For this review, take the finished solid that the model builds, in its own axes (mm). A direction names the side the tool comes from. Give positions to 0.01 mm unless a question says otherwise; leave off trailing zeros. Loops run counter-clockwise (first coordinate to the right, second up) from the corner with the lowest first, then second, coordinate; pieces in that order, holes last.
Autodesk Inventor part; units mm, degrees
ref_plane "YZ Plane" through (0, 0, 0) normal (1, 0, 0) x (0, 1, 0)
ref_plane "XZ Plane" through (0, 0, 0) normal (0, 1, 0) x (-1, 0, 0)
ref_plane "XY Plane" through (0, 0, 0) normal (0, 0, 1) x (1, 0, 0)
sketch "Sketch1" plane through (0, 0, 0) normal (0, 0, 1) x (1, 0, 0)
  line L0 (1.5, 0) -> (25.67, 0)
  line L1 (27.17, 1.5) -> (27.17, 38.5)
  line L2 (25.67, 40) -> (1.5, 40)
  line L3 (0, 38.5) -> (0, 1.5)
  arc A0 (1.5, 40) -> (0, 38.5) centre (1.5, 38.5) ccw
  arc A1 (27.17, 38.5) -> (25.67, 40) centre (25.67, 38.5) ccw
  arc A2 (25.67, 0) -> (27.17, 1.5) centre (25.67, 1.5) ccw
  arc A3 (0, 1.5) -> (1.5, 0) centre (1.5, 1.5) ccw
  point P0 (0, 0)
  point P1 (27.17, 40)
  point P2 (0, 40)
  dimension "d0" = 40
  dimension "d1" = 27.17
  dimension "d2" = 1.5
extrude "Extrusion1" add sketch "Sketch1" along normal blind 1.6
sketch "Sketch2" plane through (0, 0, 1.6) normal (0, 0, 1) x (1, 0, 0)
  line L0 (25.67, 40) -> (1.5, 40)
  line L1 (6, 40) -> (21, 40)
  line L2 (21, 40) -> (21, 25)
  line L3 (21, 25) -> (6, 25)
  line L4 (6, 25) -> (6, 40)
  line L5 (0, 38.5) -> (0, 1.5)
  line L6 (5.5, 17.5) -> (21.8, 17.5)
  line L7 (21.8, 17.5) -> (21.8, 11.8)
  line L8 (21.8, 11.8) -> (5.5, 11.8)
  line L9 (5.5, 11.8) -> (5.5, 17.5)
  line L10 (1.5, 0) -> (25.67, 0)
  line L11 (27.17, 1.5) -> (27.17, 38.5)
  line L12 (27.17, 12.8) -> (23.17, 12.8)
  line L13 (23.17, 12.8) -> (23.17, 8.8)
  line L14 (23.17, 8.8) -> (27.17, 8.8)
  line L15 (27.17, 8.8) -> (27.17, 12.8)
  point P0 (0, 0)
  dimension "d5" = 15
  dimension "d6" = 15
  dimension "d7" = 6
  dimension "d8" = 5.7
  dimension "d9" = 16.3
  dimension "d10" = 5.5
  dimension "d11" = 11.8
  dimension "d12" = 4
  dimension "d13" = 4
  dimension "d14" = 8.8
extrude "Extrusion2" add sketch "Sketch2" along normal blind 2 contours L2 L3 L4 L0
extrude "Extrusion3" add sketch "Sketch2" along normal blind 2 contours L6 L7 L8 L9
extrude "Extrusion4" add sketch "Sketch2" along normal blind 1 contours L14 L13 L12 L11
sketch "Sketch3" plane through (0, 0, 3.6) normal (0, 0, 1) x (1, 0, 0)
  line L0 (10.37, 36.1) -> (18.47, 36.1)
  line L1 (18.47, 36.1) -> (18.47, 28)
  line L2 (18.47, 28) -> (10.37, 28)
  line L3 (10.37, 28) -> (10.37, 36.1)
  line L4 (25.67, 40) -> (21, 40)
  line L5 (27.17, 12.8) -> (27.17, 38.5)
  point P0 (0, 0)
  dimension "d21" = 8.1
  dimension "d22" = 8.1
  dimension "d23" = 3.9
  dimension "d24" = 8.7
extrude "Extrusion5" add sketch "Sketch3" along normal blind 2.2
sketch "Sketch4" plane through (0, 0, 5.8) normal (0, 0, 1) x (1, 0, 0)
  circle A0 centre (14.42, 32.05) radius 3.9
  circle A1 centre (14.42, 32.05) radius 4.05
  line L0 (18.47, 36.1) -> (10.37, 36.1)
  line L1 (18.47, 28) -> (18.47, 36.1)
  point P0 (0, 0)
  dimension "d27" = 7.8
extrude "Extrusion6" add sketch "Sketch4" along normal blind 3.7 contours A0
sketch "Sketch5" plane through (0, 0, 0) normal (0, 0, -1) x (-1, 0, 0)
  line L0 (-1.035, 16.4) -> (-3.035, 16.4)
  line L1 (-3.035, 16.4) -> (-3.035, 36.4)
  line L2 (-3.035, 36.4) -> (-1.035, 36.4)
  line L3 (-1.035, 36.4) -> (-1.035, 16.4)
  line L4 (-24.135, 16.4) -> (-26.135, 16.4)
  line L5 (-26.135, 16.4) -> (-26.135, 36.4)
  line L6 (-26.135, 36.4) -> (-24.135, 36.4)
  line L7 (-24.135, 36.4) -> (-24.135, 16.4)
  line L8 (0, 38.5) -> (0, 1.5)
  line L9 (-27.17, 1.5) -> (-27.17, 38.5)
  line L10 (-1.5, 0) -> (-25.67, 0)
  line L11 (-25.67, 40) -> (-1.5, 40)
  point P0 (0, 0)
  dimension "d30" = 25.1
  dimension "d31" = 2
  dimension "d32" = 1.035
  dimension "d33" = 1.035
  dimension "d36" = 3.6
  dimension "d39" = 20
extrude "Extrusion7" add sketch "Sketch5" along normal blind 2
properties part number "esp32-cam-sp"
Q1. Mouldability with a two-part tool opening along Y and no side actions: class faces 1 (the flat face through (2, 27, -2)), 2 (the flat face through (25, 8.8, 2)), 3 (the flat face through (25, 12.8, 2)), 4 (the flat face through (14, 25, 3)) as +Y half, -Y half, draft (parallel to the pull), parting line (faces both ways), or undercut.
Answers:
face 1: draft
face 2: -Y half
face 3: +Y half
face 4: undercut
Q2. For pin 1 Ø8 at (x, y) = (13, 12.5) entering from -Z; pin 2 Ø1 at (x, z) = (24.5, -1) entering from -Y; pin 3 Ø1 at (y, z) = (35, 3) entering from -X, all flat-tipped, find the tip position at first contact; note any pin that passes through.
Answers:
pin 1: stops at z = 0
pin 2: stops at y = 16.4
pin 3: stops at x = 6
Q3. Consider section A-A on z = 2. Give the boundary of the cut face in (x, y), plus the area to 3 significant figures.
Answers:
outline: (5.5, 11.8) - (21.8, 11.8) - (21.8, 17.5) - (5.5, 17.5) - close; (6, 25) - (21, 25) - (21, 40) - (6, 40) - close; (23.17, 8.8) - (27.17, 8.8) - (27.17, 12.8) - (23.17, 12.8) - close
area: 334 mm2
Q4. Consider section C-C on x = 14.42. Give the boundary of the cut face in (y, z).
Answers:
outline: (0, 0) - (40, 0) - (40, 3.6) - (36.1, 3.6) - (36.1, 5.8) - (35.95, 5.8) - (35.95, 9.5) - (28.15, 9.5) - (28.15, 5.8) - (28, 5.8) - (28, 3.6) - (25, 3.6) - (25, 1.6) - (17.5, 1.6) - (17.5, 3.6) - (11.8, 3.6) - (11.8, 1.6) - (0, 1.6) - close
Q5. Machinability: for faces 5 (the flat face through (14, 28, 5)), 6 (the flat face through (10.37, 32, 5)), 7 (the flat face through (2, 36.4, -1)), 8 (the flat face through (26.135, 26, -1)), 9 (the cylindrical face through (16.517, 28.762, 7.624)), which of the approach directions +Z, -Z, +X, -X, +Y, -Y give a long, thin tool a straight path to every point of the face, cutting with its end or side? Answer none if there is none.
Answers:
face 5: +Z, +X, -X, -Y
face 6: +Z, -X, +Y, -Y
face 7: -Z, +X, -X, +Y
face 8: -Z, +X, +Y, -Y
face 9: +Z
Q6. Consider section D-D on y = 26. Give the boundary of the cut face in (x, z) (3 decimals), plus the area to 3 significant figures.
Answers:
outline: (0, 0) - (1.035, 0) - (1.035, -2) - (3.035, -2) - (3.035, 0) - (24.135, 0) - (24.135, -2) - (26.135, -2) - (26.135, 0) - (27.17, 0) - (27.17, 1.6) - (21, 1.6) - (21, 3.6) - (6, 3.6) - (6, 1.6) - (0, 1.6) - close
area: 81.5 mm2
Q7. For probe 1 along Y at (x, z) = (8.25, 2.75); probe 2 along X at (y, z) = (32, 6); probe 3 along Z at (x, y) = (1.5, 16), list the stretches that pass through material, from the lowest coordinate up.
Answers:
probe 1: y = 11.8 to 17.5, 25 to 40
probe 2: x = 10.52 to 18.32
probe 3: z = 0 to 1.6
Q8. Consider section B-B on y = 32.05. Give the boundary of the cut face in (x, z) (3 decimals), plus the area to 3 significant figures.
Answers:
outline: (0, 0) - (1.035, 0) - (1.035, -2) - (3.035, -2) - (3.035, 0) - (24.135, 0) - (24.135, -2) - (26.135, -2) - (26.135, 0) - (27.17, 0) - (27.17, 1.6) - (21, 1.6) - (21, 3.6) - (18.47, 3.6) - (18.47, 5.8) - (18.32, 5.8) - (18.32, 9.5) - (10.52, 9.5) - (10.52, 5.8) - (10.37, 5.8) - (10.37, 3.6) - (6, 3.6) - (6, 1.6) - (0, 1.6) - close
area: 128 mm2
